CAD build for the part. Positions are in the model's coordinates, mm. A direction names the side the tool comes from. Coordinates: 2 decimals unless noted, no trailing zeros. Loops run counter-clockwise (first coordinate to the right, second up) from the corner with the lowest first, then second, coordinate; pieces in that order, holes last.
1) Saw through at C-C, the plane y = 24.5. Write the cut outline in (x, z).
2) Saw through at B-B, the plane x = -7.25. Write the cut outline in (y, z).
3) Pin check, flat tips, straight feed: pin 1 Ø1.1 at (y, z) = (-6.5, 0) entering from +X; pin 2 Ø4 at (x, y) = (-7.5, -2) entering from +Z; pin 3 Ø3 at (x, y) = (-7.25, -5.5) entering from -Z. Stop position of each tip, or through.
4) Two-plate mould, pull along Z, no slides. Class faces 1 (the cylindrical face through (-8.21, 25.38, 0.01)), 2 (the cylindrical face through (-1.4, 16.21, -0.06)), 3 (the cylindrical face through (2, 3, 0)), 4 (the cylindrical face through (-1.4, 2.71, -0.06)): +Z half, -Z half, draft (parallel to the pull), parting line (faces both ways), or undercut.
5) Saw through at A-A, the plane z = 0. Write the cut outline in (x, y).
6) Wall check: line 1 along Y through (x, z) = (-7.25, 0.1); line 2 along Y through (x, z) = (1, -1.55); line 3 along Z through (x, y) = (0, 14.95). Give the ranges that are in metal, low to high.
7) Which spindle directions (+Z, -Z, +X, -X, +Y, -Y) get a long thin tool onto all of the face, cutting with end or side? Do faces 5 (the flat face through (0.9, 13.5, 1.3)), 6 (the flat face through (-5, 10, -0.5)), 7 (the flat face through (-4, -5, 0)), 8 (the flat face through (-4, 24, 0)). Say none if no direction does.
8) Saw through at D-D, the plane x = 0. Write the cut outline in (y, z).
```python
from build123d import *

# Parameters (mm, degrees)
SKETCH1_R           = 1.4
BOSS_EXTRUDE1_DEPTH = 5.5
SKETCH2_R           = 1.4
BOSS_EXTRUDE2_DEPTH = 5.5
SKETCH3_W           = 8
SKETCH3_H           = 1
BOSS_EXTRUDE3_DEPTH = 13.5
SKETCH4_W           = 6.5
SKETCH4_H           = 1
BOSS_EXTRUDE4_DEPTH = 9.5
SKETCH5_W           = 6.5
SKETCH5_H           = 1
BOSS_EXTRUDE5_DEPTH = 9.5
FILLET1_R           = 0.5
CUT_EXTRUDE1_REACH  = 4.5
SKETCH6_R           = 1.303868107


with BuildPart() as part:
    # Sketch1 → Boss-Extrude1 (new body)
    with BuildSketch(Plane(origin=(0, 0, 0), x_dir=(1, 0, 0), z_dir=(0, 1, 0))):
        with BuildLine():
            Line((-1.936491673, 0.5), (-10.5, 0.5))
            Line((-10.5, 0.5), (-10.5, -0.5))
            Line((-10.5, -0.5), (-1.936491673, -0.5))
            ThreePointArc((-1.936491673, -0.5), (2, 0), (-1.936491673, 0.5))
        make_face()
        Circle(SKETCH1_R, mode=Mode.SUBTRACT)
    extrude(amount=BOSS_EXTRUDE1_DEPTH)



with BuildPart() as body_2:
    # Sketch2 → Boss-Extrude2 (new body)
    with BuildSketch(Plane(origin=(0, 13.5, 0), x_dir=(1, 0, 0), z_dir=(0, 1, 0))):
        with BuildLine():
            Line((-1.936491673, 0.5), (-10.5, 0.5))
            Line((-10.5, 0.5), (-10.5, -0.5))
            Line((-10.5, -0.5), (-1.936491673, -0.5))
            ThreePointArc((-1.936491673, -0.5), (2, 0), (-1.936491673, 0.5))
        make_face()
        Circle(SKETCH2_R, mode=Mode.SUBTRACT)
    extrude(amount=BOSS_EXTRUDE2_DEPTH)


with BuildPart() as part_1:
    add(part.part)

    add(body_2.part)  # Boss-Extrude3 merges body 2
    # Sketch3 → Boss-Extrude3 (add)
    with BuildSketch(Plane(origin=(0, 5.5, 0), x_dir=(1, 0, 0), z_dir=(0, 1, 0))):
        with Locations((-6.5, 0)):
            Rectangle(SKETCH3_W, SKETCH3_H)
    extrude(amount=BOSS_EXTRUDE3_DEPTH)

    # Sketch4 → Boss-Extrude4 (add)
    with BuildSketch(Plane(origin=(0, 19, 0), x_dir=(1, 0, 0), z_dir=(0, 1, 0))):
        with Locations((-7.25, 0)):
            Rectangle(SKETCH4_W, SKETCH4_H)
    extrude(amount=BOSS_EXTRUDE4_DEPTH)

    # Sketch5 → Boss-Extrude5 (add)
    with BuildSketch(Plane.XZ):
        with Locations((-7.25, 0)):
            Rectangle(SKETCH5_W, SKETCH5_H)
    extrude(amount=BOSS_EXTRUDE5_DEPTH)

    # Fillet1
    fillet1_edges = [part_1.edges().sort_by_distance(p)[0] for p in [
        (-2.5, 13.5, 0),
        (-2.5, 5.5, 0),
    ]]
    fillet(fillet1_edges, radius=FILLET1_R)

    # Sketch6 → Cut-Extrude1 (cut, up to next)
    with BuildSketch(Plane.XY.offset(0.5), mode=Mode.PRIVATE) as cut_extrude1_sk1:
        with Locations((-7.25, -5.5)):
            Circle(SKETCH6_R)
    cut_extrude1_tool1 = extrude(cut_extrude1_sk1.sketch, amount=-CUT_EXTRUDE1_REACH, mode=Mode.PRIVATE) & part_1.part
    add(cut_extrude1_tool1.solids().sort_by_distance((-7.25, -5.5, 0.5))[0], mode=Mode.SUBTRACT)
    # Sketch6 → Cut-Extrude1 (cut, up to next)
    with BuildSketch(Plane.XY.offset(0.5), mode=Mode.PRIVATE) as cut_extrude1_sk2:
        with Locations((-7.25, 9.5)):
            Circle(SKETCH6_R)
    cut_extrude1_tool2 = extrude(cut_extrude1_sk2.sketch, amount=-CUT_EXTRUDE1_REACH, mode=Mode.PRIVATE) & part_1.part
    add(cut_extrude1_tool2.solids().sort_by_distance((-7.25, 9.5, 0.5))[0], mode=Mode.SUBTRACT)
    # Sketch6 → Cut-Extrude1 (cut, up to next)
    with BuildSketch(Plane.XY.offset(0.5), mode=Mode.PRIVATE) as cut_extrude1_sk3:
        with Locations((-7.25, 24.5)):
            Circle(SKETCH6_R)
    cut_extrude1_tool3 = extrude(cut_extrude1_sk3.sketch, amount=-CUT_EXTRUDE1_REACH, mode=Mode.PRIVATE) & part_1.part
    add(cut_extrude1_tool3.solids().sort_by_distance((-7.25, 24.5, 0.5))[0], mode=Mode.SUBTRACT)


solid = part_1.part
```
Data:
1. outline: (-10.5, -0.5) - (-8.55, -0.5) - (-8.55, 0.5) - (-10.5, 0.5) - close; (-5.95, -0.5) - (-4, -0.5) - (-4, 0.5) - (-5.95, 0.5) - close
2. outline: (-9.5, -0.5) - (-6.8, -0.5) - (-6.8, 0.5) - (-9.5, 0.5) - close; (-4.2, -0.5) - (8.2, -0.5) - (8.2, 0.5) - (-4.2, 0.5) - close; (10.8, -0.5) - (23.2, -0.5) - (23.2, 0.5) - (10.8, 0.5) - close; (25.8, -0.5) - (28.5, -0.5) - (28.5, 0.5) - (25.8, 0.5) - close
3. pin 1: stops at x = -4
3. pin 2: stops at z = 0.5
3. pin 3: stops at z = -0.5
4. face 1: draft
4. face 2: undercut
4. face 3: parting line
4. face 4: undercut
5. outline: (-10.5, -9.5) - (-4, -9.5) - (-4, 0) - (-1.4, 0) - (-1.4, 5.5) - (-2, 5.5) arc R0.5 cw to (-2.5, 6) - (-2.5, 13) arc R0.5 cw to (-2, 13.5) - (-1.4, 13.5) - (-1.4, 19) - (-4, 19) - (-4, 28.5) - (-10.5, 28.5) - close; (1.4, 0) - (2, 0) - (2, 5.5) - (1.4, 5.5) - close; (1.4, 13.5) - (2, 13.5) - (2, 19) - (1.4, 19) - close; hole circle Ø2.61 at (-7.25, -5.5); hole circle Ø2.61 at (-7.25, 9.5); hole circle Ø2.61 at (-7.25, 24.5)
6. line 1: y = -9.5 to -6.8, -4.2 to 8.2, 10.8 to 23.2, 25.8 to 28.5
6. line 2: y = 0 to 5.5, 13.5 to 19
6. line 3: z = -2 to -1.4, 1.4 to 2
7. face 5: +Z, -Z, +X
7. face 6: -Z, -X, +Y, -Y
7. face 7: +Z, -Z, +X, -Y
7. face 8: +Z, -Z, +X, +Y
8. outline: (0, -2) - (5.5, -2) - (5.5, -1.4) - (0, -1.4) - close; (0, 1.4) - (5.5, 1.4) - (5.5, 2) - (0, 2) - close; (13.5, -2) - (19, -2) - (19, -1.4) - (13.5, -1.4) - close; (13.5, 1.4) - (19, 1.4) - (19, 2) - (13.5, 2) - close
